```python
from build123d import *

# Parameters (mm, degrees)
F0_W     = 110
F0_H     = 110
F0_W_2   = 106
F0_H_2   = 106
F1_DEPTH = 3
F2_DEPTH = 7
F3_DEPTH = 7


with BuildPart() as f1:
    # F0 (on Top) → F1 (new body)
    with BuildSketch(Plane.XY):
        with BuildLine():
            Line((60.5, -53.5089111648), (60.5, 54))
            ThreePointArc((60.5, 54), (58.5961940777, 58.5961940777), (54, 60.5))
            Line((54, 60.5), (-53.5089111648, 60.5))
            ThreePointArc((-53.5089111648, 60.5), (-58.452357488, 58.452357488), (-60.5, 53.5089111648))
            Line((-60.5, 53.5089111648), (-60.5, -54))
            ThreePointArc((-60.5, -54), (-58.5961940777, -58.5961940777), (-54, -60.5))
            Line((-54, -60.5), (53.5089111648, -60.5))
            ThreePointArc((53.5089111648, -60.5), (58.452357488, -58.452357488), (60.5, -53.5089111648))
        make_face()
        with BuildLine():
            ThreePointArc((-59, 53.5089111648), (-57.3916978342, 57.3916967983), (-53.5089126297, 59))
            Line((-53.5089126297, 59), (54, 59))
            ThreePointArc((54, 59), (57.5355339059, 57.5355339059), (59, 54))
            Line((59, 54), (59, -53.5089111648))
            ThreePointArc((59, -53.5089111648), (57.3916973163, -57.3916973163), (53.5089111648, -59))
            Line((53.5089111648, -59), (-54, -59))
            ThreePointArc((-54, -59), (-57.535533861, -57.5355339509), (-59, -54.0000001272))
            Line((-59, -54.0000001272), (-59, 53.5089111648))
        make_face(mode=Mode.SUBTRACT)
        with BuildLine():
            Line((54, 59), (-53.5089126297, 59))
            ThreePointArc((-53.5089126297, 59), (-57.3916978342, 57.3916967983), (-59, 53.5089111648))
            Line((-59, 53.5089111648), (-59, -54.0000001272))
            ThreePointArc((-59, -54.0000001272), (-57.535533861, -57.5355339509), (-54, -59))
            Line((-54, -59), (53.5089111648, -59))
            ThreePointArc((53.5089111648, -59), (57.3916973163, -57.3916973163), (59, -53.5089111648))
            Line((59, -53.5089111648), (59, 54))
            ThreePointArc((59, 54), (57.5355339059, 57.5355339059), (54, 59))
        make_face()
        Rectangle(F0_W, F0_H, mode=Mode.SUBTRACT)
        Rectangle(F0_W_2, F0_H_2)
        Polygon((-53, -53), (-55, -55), (55, -55), (53, -53), align=None)
        Polygon((-53, 53), (-55, 55), (-55, -55), (-53, -53), align=None)
        Polygon((55, 55), (-55, 55), (-53, 53), (53, 53), align=None)
        Polygon((55, -55), (55, 55), (53, 53), (53, -53), align=None)
    extrude(amount=F1_DEPTH)

    # F0 (on Top) → F2 (join)
    with BuildSketch(Plane.XY):
        with BuildLine():
            Line((60.5, -53.5089111648), (60.5, 54))
            ThreePointArc((60.5, 54), (58.5961940777, 58.5961940777), (54, 60.5))
            Line((54, 60.5), (-53.5089111648, 60.5))
            ThreePointArc((-53.5089111648, 60.5), (-58.452357488, 58.452357488), (-60.5, 53.5089111648))
            Line((-60.5, 53.5089111648), (-60.5, -54))
            ThreePointArc((-60.5, -54), (-58.5961940777, -58.5961940777), (-54, -60.5))
            Line((-54, -60.5), (53.5089111648, -60.5))
            ThreePointArc((53.5089111648, -60.5), (58.452357488, -58.452357488), (60.5, -53.5089111648))
        make_face()
        with BuildLine():
            ThreePointArc((-59, 53.5089111648), (-57.3916978342, 57.3916967983), (-53.5089126297, 59))
            Line((-53.5089126297, 59), (54, 59))
            ThreePointArc((54, 59), (57.5355339059, 57.5355339059), (59, 54))
            Line((59, 54), (59, -53.5089111648))
            ThreePointArc((59, -53.5089111648), (57.3916973163, -57.3916973163), (53.5089111648, -59))
            Line((53.5089111648, -59), (-54, -59))
            ThreePointArc((-54, -59), (-57.535533861, -57.5355339509), (-59, -54.0000001272))
            Line((-59, -54.0000001272), (-59, 53.5089111648))
        make_face(mode=Mode.SUBTRACT)
    extrude(amount=F2_DEPTH)

    # F0 (on Top) → F3 (join)
    with BuildSketch(Plane.XY):
        Polygon((55, 55), (-55, 55), (-53, 53), (53, 53), align=None)
        Polygon((-53, -53), (-55, -55), (55, -55), (53, -53), align=None)
        Polygon((-53, 53), (-55, 55), (-55, -55), (-53, -53), align=None)
        Polygon((55, -55), (55, 55), (53, 53), (53, -53), align=None)
    extrude(amount=F3_DEPTH)


solid = f1.part
```
Source: CAD feature listing. Evaluate the final solid. Frame: model axes, mm. A direction names the side the tool comes from. Give positions to 0.01 mm unless a question says otherwise; leave off trailing zeros. Order: outer loops, then holes, each group sorted by start corner. A loop starts at its lowest first (then second) coordinate and runs counter-clockwise, first axis right, second up. Notation, with made-up numbers: (71.25, -30) -> (118.25, -30) arc R14 cw to (118.25, -11) -> close; hole circle Ø2 at (-20, 23.25). An arc over 180 degrees is marked (long way). Use a Markdown table: item, result.
Q1. Material intervals for line 1 (X direction, y = 28, z = 4); line 2 (Z direction, x = 16, y = -26.5), sorted ascending. Write a range as [from, to].
A:
| item | result |
|---|---|
| line 1 | [-60.5, -59], [-55, -53], [53, 55], [59, 60.5] |
| line 2 | [0, 3] |
Q2. Section A-A (x = 51). Return the cut outline in (y, z).
A:
| item | result |
|---|---|
| outline | (-60.5, 0) -> (60.5, 0) -> (60.5, 7) -> (59, 7) -> (59, 3) -> (55, 3) -> (55, 7) -> (53, 7) -> (53, 3) -> (-53, 3) -> (-53, 7) -> (-55, 7) -> (-55, 3) -> (-59, 3) -> (-59, 7) -> (-60.5, 7) -> close |
Q3. First-contact query: P1, Ø6, axis at x = -26, y = -33, coming from the +Z side. Flat tip, straight axial feed; report the tip coordinate or a pass-through.
A:
| item | result |
|---|---|
| P1 | z = 3 |
Q4. Pull-direction query (Y, two-part tool) for faces 1 (the face through (-59, -1, 5)), 2 (the face through (60.5, -1, 3)), 3 (the face through (58.398, -58.506, 3.451)); classes: +Y half, -Y half, draft (parallel to the pull), parting line (faces both ways), or undercut.
A:
| item | result |
|---|---|
| face 1 | undercut |
| face 2 | draft |
| face 3 | -Y half |
Q5. Access query for faces 4 (the face through (-1, 1, 0)), 5 (the face through (53, 1, 5)). Directions: +Z, -Z, +X, -X, +Y, -Y. A direction counts if a zero-diameter tool reaches every point of the face in a straight line with its end or side. Return the directions, or none.
A:
| item | result |
|---|---|
| face 4 | -Z, +X, -X, +Y, -Y |
| face 5 | +Z |
